from build123d import *

# Parameters (mm, degrees)
CROQUIS3_W              = 7.5
CROQUIS3_H              = 15
SALIENTE_EXTRUIR1_DEPTH = 3
CROQUIS4_R              = 1.5
CROQUIS4_W              = 14
CROQUIS4_H              = 45
CROQUIS4_W_2            = 10
CROQUIS4_H_2            = 3
CORTAR_EXTRUIR1_DEPTH   = 3
SALIENTE_EXTRUIR2_DEPTH = 3
REDONDEO2_R             = 0.25
REDONDEO3_R             = 1
CROQUIS6_R              = 1.5
CROQUIS6_W              = 5
CROQUIS6_H              = 5
CROQUIS6_W_2            = 10
CROQUIS6_H_2            = 4
CORTAR_EXTRUIR2_DEPTH   = 5
CROQUIS7_R              = 1.5
CORTAR_EXTRUIR4_DEPTH   = 5


with BuildPart() as part:
    # Croquis3 → Saliente-Extruir1 (new body)
    with BuildSketch(Plane(origin=(0, 0, 0), x_dir=(1, 0, 0), z_dir=(0, 1, 0))):
        with BuildLine():
            Line((-50, -45), (50, -45))
            Line((50, -45), (50, 28.189923373))
            Line((50, 28.189923373), (56.6, 28.189923373))
            ThreePointArc((56.6, 28.189923373), (58.367766953, 28.92215642), (59.1, 30.689923373))
            Line((59.1, 30.689923373), (59.1, 38.189923373))
            Line((59.1, 38.189923373), (56.1, 38.189923373))
            Line((56.1, 38.189923373), (56.1, 33.189923373))
            Line((56.1, 33.189923373), (53.1, 33.189923373))
            Line((53.1, 33.189923373), (53.1, 38.189923373))
            Line((53.1, 38.189923373), (50.1, 38.189923373))
            Line((50.1, 38.189923373), (50.1, 43.139923373))
            ThreePointArc((50.1, 43.139923373), (49.605586306, 44.632445926), (48.317901143, 45.534629607))
            Line((48.317901143, 45.534629607), (0.615531773, 59.835166775))
            ThreePointArc((0.615531773, 59.835166775), (0, 59.908733938), (-0.615531773, 59.835166775))
            Line((-0.615531773, 59.835166775), (-48.317901143, 45.534629607))
            ThreePointArc((-48.317901143, 45.534629607), (-49.605586306, 44.632445926), (-50.1, 43.139923373))
            Line((-50.1, 43.139923373), (-50.1, 38.189923373))
            Line((-50.1, 38.189923373), (-53.1, 38.189923373))
            Line((-53.1, 38.189923373), (-53.1, 33.189923373))
            Line((-53.1, 33.189923373), (-56.1, 33.189923373))
            Line((-56.1, 33.189923373), (-56.1, 38.189923373))
            Line((-56.1, 38.189923373), (-59.1, 38.189923373))
            Line((-59.1, 38.189923373), (-59.1, 30.689923373))
            ThreePointArc((-59.1, 30.689923373), (-58.367766953, 28.92215642), (-56.6, 28.189923373))
            Line((-56.6, 28.189923373), (-50, 28.189923373))
            Line((-50, 28.189923373), (-50, -45))
        make_face()
        with Locations((28.75, 0)):
            Rectangle(CROQUIS3_W, CROQUIS3_H, mode=Mode.SUBTRACT)
        with Locations((-28.75, 0)):
            Rectangle(CROQUIS3_W, CROQUIS3_H, mode=Mode.SUBTRACT)
        Polygon((-23.595339952, 49.778243466), (-18.595339952, 51.277177099), (-17.695979772, 48.277177099), (-27.695979772, 45.279309832), (-28.595339952, 48.279309832), align=None, mode=Mode.SUBTRACT)
        Polygon((28.595339952, 48.279309832), (27.695979772, 45.279309832), (17.695979772, 48.277177099), (18.595339952, 51.277177099), (23.595339952, 49.778243466), align=None, mode=Mode.SUBTRACT)
    extrude(amount=SALIENTE_EXTRUIR1_DEPTH)

    # Croquis4 → Cortar-Extruir1 (cut, symmetric)
    with BuildSketch(Plane(origin=(0, 3, 0), x_dir=(1, 0, 0), z_dir=(0, 1, 0))):
        with Locations(Location((0.25, -38.703289419, 0), (0, 0, 270))):
            Circle(CROQUIS4_R)
        with Locations(Location((-39, 9, 0), (0, 0, 270))):
            Circle(CROQUIS4_R)
        with Locations(Location((39, 9, 0), (0, 0, 270))):
            Circle(CROQUIS4_R)
        with Locations(Location((39, -9, 0), (0, 0, 270))):
            Circle(CROQUIS4_R)
        with Locations(Location((-39, -9, 0), (0, 0, 270))):
            Circle(CROQUIS4_R)
        with Locations(Location((-43.980956203, -38.703289419, 0), (0, 0, 270))):
            Circle(CROQUIS4_R)
        with Locations(Location((-13.25, -38.703289419, 0), (0, 0, 270))):
            Circle(CROQUIS4_R)
        with Locations(Location((13.25, -38.703289419, 0), (0, 0, 270))):
            Circle(CROQUIS4_R)
        with Locations(Location((43.980956203, -38.703289419, 0), (0, 0, 270))):
            Circle(CROQUIS4_R)
        with Locations((51.75, -0.930038314)):
            Rectangle(CROQUIS4_W, CROQUIS4_H)
        with Locations((-51.75, -0.930038314)):
            Rectangle(CROQUIS4_W, CROQUIS4_H)
        with Locations((-33, -43.5)):
            Rectangle(CROQUIS4_W_2, CROQUIS4_H_2)
        with Locations((33, -43.5)):
            Rectangle(CROQUIS4_W_2, CROQUIS4_H_2)
    extrude(amount=CORTAR_EXTRUIR1_DEPTH, both=True, mode=Mode.SUBTRACT)

    # Croquis5 → Saliente-Extruir2 (add)
    with BuildSketch(Plane(origin=(0, 0, 0), x_dir=(1, 0, 0), z_dir=(0, 1, 0))):
        with BuildLine():
            Line((-50, -45), (50, -45))
            Line((50, -45), (50, -45.5))
            ThreePointArc((50, -45.5), (49.267766953, -47.267766953), (47.5, -48))
            Line((47.5, -48), (-47.5, -48))
            ThreePointArc((-47.5, -48), (-49.267766953, -47.267766953), (-50, -45.5))
            Line((-50, -45.5), (-50, -45))
        make_face()
    extrude(amount=SALIENTE_EXTRUIR2_DEPTH)

    # Redondeo2
    redondeo2_edges = [part.edges().sort_by_distance(p)[0] for p in [
        (-44.75, 1.5, -21.569961686),
        (-44.75, 1.5, 23.430038314),
        (44.75, 1.5, 23.430038314),
        (44.75, 1.5, -21.569961686),
        (-56.1, 1.5, -38.189923373),
        (-56.1, 1.5, -33.189923373),
        (-53.1, 1.5, -33.189923373),
        (-53.1, 1.5, -38.189923373),
        (53.1, 1.5, -38.189923373),
        (53.1, 1.5, -33.189923373),
        (56.1, 1.5, -33.189923373),
        (56.1, 1.5, -38.189923373),
    ]]
    fillet(redondeo2_edges, radius=REDONDEO2_R)

    # Redondeo3
    redondeo3_edges = [part.edges().sort_by_distance(p)[0] for p in [
        (-50, 1.5, -21.569961686),
        (-50, 1.5, 23.430038314),
        (50, 1.5, -21.569961686),
        (50, 1.5, 23.430038314),
        (-59.1, 1.5, -38.189923373),
        (-50.1, 1.5, -38.189923373),
        (50.1, 1.5, -38.189923373),
        (59.1, 1.5, -38.189923373),
    ]]
    fillet(redondeo3_edges, radius=REDONDEO3_R)

    # Croquis6 → Cortar-Extruir2 (cut, symmetric)
    with BuildSketch(Plane(origin=(0, 3, 0), x_dir=(1, 0, 0), z_dir=(0, 1, 0))):
        with Locations(Location((-18.777873171, -25.555868596, 0), (0, 0, 270))):
            Circle(CROQUIS6_R)
        with Locations(Location((-18.777873171, 38.444131404, 0), (0, 0, 270))):
            Circle(CROQUIS6_R)
        with Locations(Location((19.222126829, -25.555868596, 0), (0, 0, 270))):
            Circle(CROQUIS6_R)
        with Locations(Location((19.222126829, 38.444131404, 0), (0, 0, 270))):
            Circle(CROQUIS6_R)
        with Locations((-28.75, 13)):
            Rectangle(CROQUIS6_W, CROQUIS6_H)
        with Locations((0.222126829, -25.555868596)):
            Rectangle(CROQUIS6_W_2, CROQUIS6_H_2)
    extrude(amount=CORTAR_EXTRUIR2_DEPTH, both=True, mode=Mode.SUBTRACT)

    # Croquis7 → Cortar-Extruir4 (cut, symmetric)
    with BuildSketch(Plane(origin=(0, 3, 0), x_dir=(1, 0, 0), z_dir=(0, 1, 0))):
        with Locations(Location((29.022405425, 27.963870269, 0), (0, 0, 270))):
            Circle(CROQUIS7_R)
        with Locations(Location((-29, -16.050530834, 0), (0, 0, 270))):
            Circle(CROQUIS7_R)
        with Locations(Location((29, -16.050530834, 0), (0, 0, 270))):
            Circle(CROQUIS7_R)
        with Locations(Location((-28.977594575, 27.963870269, 0), (0, 0, 270))):
            Circle(CROQUIS7_R)
        with Locations(Location((-10.977594575, 44.444131404, 0), (0, 0, 270))):
            Circle(CROQUIS7_R)
        with Locations(Location((11.022405425, 44.444131404, 0), (0, 0, 270))):
            Circle(CROQUIS7_R)
        with Locations(Location((0, 38.444131404, 0), (0, 0, 270))):
            Circle(CROQUIS7_R)
    extrude(amount=CORTAR_EXTRUIR4_DEPTH, both=True, mode=Mode.SUBTRACT)


solid = part.part
Geometry check sheet. Reference: the model listing, model coordinates, mm. A direction names the side the tool comes from. Round coordinates to 2 decimals unless told otherwise and drop trailing zeros. Order: outer loops, then holes, each group sorted by start corner. A loop starts at its lowest first (then second) coordinate and runs counter-clockwise, first axis right, second up. Notation, with made-up numbers: M -10,88 L 42,88 A9 cw 42,92 Z; hole C 82.25,19.5 d11. An arc over 180 degrees is marked long. Answer in a Markdown table with one row per item. Add a question column.
Item 1: Material ranges on L1, parallel to X at y = 1.5, z = -36.5; L2, parallel to X at y = 0.3, z = 4; L3, parallel to Z at x = -30, y = 1.15, recorded low to high. Write a range as [from, to].
Item 2: Set-up check for faces 1 (the face through (24.801, 1.479, -52.585)), 2 (the face through (55, 1, -33.19)), 3 (the face through (-53, 1, -28.19)), 4 (the face through (-50.1, 1, -41)), 5 (the face through (29, 1, 7.5)): record each of +Z, -Z, +X, -X, +Y, -Y from which the full face is reachable in a straight line by a thin tool's end or side.
Item 3: Sectioned sample at A-A, the plane z = 5.5. Enter the section's corners in (x, y), plus the area to 4 significant figures.
Item 4: Draft check along X on faces 6 (the face through (-10.912, 1.521, -45.943)), 7 (the face through (-59.1, 1, -34)), 8 (the face through (50, 1, -25)). Enter one of: released by +X, released by -X, zero draft, split by the parting line, or undercut.
Item 5: Sectioned sample at C-C, the plane x = 34. Enter the section's corners in (y, z), plus the area to 3 significant figures.
Item 6: Depth check by flat-ended pin: pin 1 Ø1.5 at (y, z) = (1.5, 43.5) entering from +X; pin 2 Ø0.9 at (x, y) = (-32.5, 1) entering from -Z; pin 3 Ø0.9 at (x, y) = (29, 2) entering from -Z. Enter the tip coordinate at first touch or a pass-through.
Item 7: Sectioned sample at B-B, the plane z = -12. Enter the section's corners in (x, y), plus the area to 4 significant figures.
Filled in:
| question | item | result |
|---|---|---|
| 1 | L1 | x = [-59.1, -56.1], [-53.1, 53.1], [56.1, 59.1] |
| 1 | L2 | x = [-44.75, -32.5], [-25, 25], [32.5, 44.75] |
| 1 | L3 | z = [-51.03, -29.06], [-26.87, -15.5], [-10.5, -7.5], [7.5, 14.93], [17.17, 42], [45, 48] |
| 2 | face 1 | -Z, +X, +Y, -Y |
| 2 | face 2 | -Z, +Y, -Y |
| 2 | face 3 | +Z, -X, +Y, -Y |
| 2 | face 4 | -Z, -X, +Y, -Y |
| 2 | face 5 | +Y, -Y |
| 3 | outline | M -44.75,0 L -32.5,0 L -32.5,3 L -44.75,3 Z; M -25,0 L 25,0 L 25,3 L -25,3 Z; M 32.5,0 L 44.75,0 L 44.75,3 L 32.5,3 Z |
| 3 | area | 223.5 mm² |
| 4 | face 6 | undercut |
| 4 | face 7 | released by -X |
| 4 | face 8 | released by +X |
| 5 | outline | M 0,-49.83 L 3,-49.83 L 3,42 L 0,42 Z; M 0,45 L 3,45 L 3,48 L 0,48 Z |
| 5 | area | 284 mm² |
| 6 | pin 1 | stops at x = 50 |
| 6 | pin 2 | stops at z = -50.41 |
| 6 | pin 3 | stops at z = -51.46 |
| 7 | outline | M -44.75,0 L -31.25,0 L -31.25,3 L -44.75,3 Z; M -26.25,0 L 44.75,0 L 44.75,3 L -26.25,3 Z |
| 7 | area | 253.5 mm² |
